from build123d import *

# Parameters (mm, degrees)
BOSS_EXTRUDE1_DEPTH = 3


with BuildPart() as part:
    # Sketch1 → Boss-Extrude1 (new body)
    with BuildSketch(Plane(origin=(0, 0, 0), x_dir=(1, 0, 0), z_dir=(0, 1, 0))):
        Polygon((-65, -65), (-57.5, -65), (-57.5, -61), (-47.5, -61), (-47.5, -65), (-32.5, -65), (-32.5, -61), (-22.5, -61), (-22.5, -65), (-7.5, -65), (-7.5, -61), (7.5, -61), (7.5, -65), (22.5, -65), (22.5, -61), (32.5, -61), (32.5, -65), (47.5, -65), (47.5, -61), (57.5, -61), (57.5, -65), (65, -65), (65, -57.5), (61, -57.5), (61, -47.5), (65, -47.5), (65, -32.5), (61, -32.5), (61, -22.5), (65, -22.5), (65, -7.5), (61, -7.5), (61, 7.5), (65, 7.5), (65, 22.5), (61, 22.5), (61, 32.5), (65, 32.5), (65, 47.5), (61, 47.5), (61, 57.5), (65, 57.5), (65, 65), (57.5, 65), (57.5, 61), (47.5, 61), (47.5, 65), (32.5, 65), (32.5, 61), (22.5, 61), (22.5, 65), (7.5, 65), (7.5, 61), (-7.5, 61), (-7.5, 65), (-22.5, 65), (-22.5, 61), (-32.5, 61), (-32.5, 65), (-47.5, 65), (-47.5, 61), (-57.5, 61), (-57.5, 65), (-65, 65), (-65, 57.5), (-61, 57.5), (-61, 47.5), (-65, 47.5), (-65, 32.5), (-61, 32.5), (-61, 22.5), (-65, 22.5), (-65, 7.5), (-61, 7.5), (-61, -7.5), (-65, -7.5), (-65, -22.5), (-61, -22.5), (-61, -32.5), (-65, -32.5), (-65, -47.5), (-61, -47.5), (-61, -57.5), (-65, -57.5), align=None)
        with BuildLine():
            Line((-37.5, 50), (-37.5, -50))
            ThreePointArc((-37.5, -50), (-40, -52.5), (-42.5, -50))
            Line((-42.5, -50), (-42.5, 50))
            ThreePointArc((-42.5, 50), (-40, 52.5), (-37.5, 50))
        make_face(mode=Mode.SUBTRACT)
        with BuildLine():
            Line((-12.5, 50), (-12.5, -50))
            ThreePointArc((-12.5, -50), (-15, -52.5), (-17.5, -50))
            Line((-17.5, -50), (-17.5, 50))
            ThreePointArc((-17.5, 50), (-15, 52.5), (-12.5, 50))
        make_face(mode=Mode.SUBTRACT)
        with BuildLine():
            Line((37.5, 50), (37.5, -50))
            ThreePointArc((37.5, -50), (40, -52.5), (42.5, -50))
            Line((42.5, -50), (42.5, 50))
            ThreePointArc((42.5, 50), (40, 52.5), (37.5, 50))
        make_face(mode=Mode.SUBTRACT)
        with BuildLine():
            Line((12.5, 50), (12.5, -50))
            ThreePointArc((12.5, -50), (15, -52.5), (17.5, -50))
            Line((17.5, -50), (17.5, 50))
            ThreePointArc((17.5, 50), (15, 52.5), (12.5, 50))
        make_face(mode=Mode.SUBTRACT)
    extrude(amount=BOSS_EXTRUDE1_DEPTH)


solid = part.part
Source: CAD feature listing. Evaluate the final solid. Frame: model axes, mm. A direction names the side the tool comes from. Coordinates: 2 decimals unless noted, no trailing zeros. Loops run counter-clockwise (first coordinate to the right, second up) from the corner with the lowest first, then second, coordinate; pieces in that order, holes last. Notation, with made-up numbers: (71.5, 9.5) - (84.5, 9.5) arc R18 cw to (84.5, 37.5) - close; hole circle Ø4 at (61, -7). An arc over 180 degrees is marked (long way). One line per item, written item: value. Start each with the question number.
1. Mould query, pull axis Z, two halves, no side actions, for faces 5 (the flat face through (61, 1, -65)), 6 (the flat face through (40, 1, 65)), 7 (the cylindrical face through (-15.1, 1.5, -52.5)). Classes: pulls with the +Z half, pulls with the -Z half, needs draft (parallel to the pull), parting line crosses it, or undercut.
2. Ray query, L1, parallel to X at y = 1.75, z = -23; L2, parallel to X at y = 0.2, z = 37; L3, parallel to Z at x = -40, y = 1. Return the intervals inside material, ascending.
3. Contact query for flat-ended pins moving along their axis: P1, Ø1.5, axis at x = 53.5, y = 1.5, coming from the +Z side; P2, Ø1.5, axis at y = 1, z = 29.5, coming from the -X side; P3, Ø1.5, axis at x = 54.5, y = 1, coming from the -Z side; P4, Ø4, axis at x = -11.5, z = -17, coming from the -Y side. Output: stop coordinate, or through.
4. Section B-B (x = -40). Return the cut outline in (y, z), and give its area (3 significant figures).
5. Set-up query: faces 1 (the flat face through (-37.5, 1, -1)), 2 (the flat face through (-52, 1, -61)), 3 (the flat face through (63, 1, -7.5)), 4 (the flat face through (-63, 1, -22.5)). Return all of +Z, -Z, +X, -X, +Y, -Y with unobstructed straight access to the full face (end or side cutting, diameter ignored); none if empty.
6. Section C-C (y = 0.85). State how many separate pieces and enclosed holes the cut face has, and give its area (3 significant figures).
7. Section A-A (z = -45). Return the cut outline in (x, y).
8. Section D-D (x = 2). Return the cut outline in (y, z).
Verdict:
1. face 5: pulls with the -Z half
1. face 6: pulls with the +Z half
1. face 7: undercut
2. L1: x = -61 to -42.5, -37.5 to -17.5, -12.5 to 12.5, 17.5 to 37.5, 42.5 to 61
2. L2: x = -65 to -42.5, -37.5 to -17.5, -12.5 to 12.5, 17.5 to 37.5, 42.5 to 65
2. L3: z = -65 to -52.5, 52.5 to 65
3. P1: stops at z = 61
3. P2: stops at x = -61
3. P3: stops at z = -61
3. P4: stops at y = 0
4. outline: (0, -65) - (3, -65) - (3, -52.5) - (0, -52.5) - close; (0, 52.5) - (3, 52.5) - (3, 65) - (0, 65) - close
4. area: 75.0 mm2
5. face 1: +Y, -Y
5. face 2: -Z, +Y, -Y
5. face 3: +X, +Y, -Y
5. face 4: -X, +Y, -Y
6. separate pieces: 1
6. enclosed holes: 4
6. area: 13,900 mm2
7. outline: (-65, 0) - (-42.5, 0) - (-42.5, 3) - (-65, 3) - close; (-37.5, 0) - (-17.5, 0) - (-17.5, 3) - (-37.5, 3) - close; (-12.5, 0) - (12.5, 0) - (12.5, 3) - (-12.5, 3) - close; (17.5, 0) - (37.5, 0) - (37.5, 3) - (17.5, 3) - close; (42.5, 0) - (65, 0) - (65, 3) - (42.5, 3) - close
8. outline: (0, -61) - (3, -61) - (3, 61) - (0, 61) - close
